Design review of the part built by this model. Coordinates are the model's own, in mm. A direction names the side the tool comes from. Round coordinates to 2 decimals unless told otherwise and drop trailing zeros. Order: outer loops, then holes, each group sorted by start corner. A loop starts at its lowest first (then second) coordinate and runs counter-clockwise, first axis right, second up. Notation, with made-up numbers: (-17.75, -3) - (36.25, -3) arc R28 ccw to (36.25, 34) - close; hole circle Ø3 at (-35.5, 7.5). An arc over 180 degrees is marked (long way). Write item = value, one per line.
from build123d import *

# Parameters (mm, degrees)
BOSS_EXTRUDE1_DEPTH = 60
BOSS_EXTRUDE2_DEPTH = 1.5
CUT_EXTRUDE1_DEPTH  = 122.5
FILLET1_R           = 2
SKETCH4_R           = 1
CUT_EXTRUDE2_DEPTH  = 122.5
SKETCH5_W           = 20.552185026
SKETCH5_H           = 10
CUT_EXTRUDE3_DEPTH  = 66.5
CHAMFER2_SIZE       = 4


with BuildPart() as part:
    # Sketch1 → Boss-Extrude1 (new body)
    with BuildSketch(Plane(origin=(0, 0, 0), x_dir=(1, 0, 0), z_dir=(0, 1, 0))):
        Polygon((-25.683056898, 37.455662838), (17.724607753, 43.304991821), (29.01282847, -40.464497095), (-14.394836181, -46.313826078), align=None)
        Polygon((-23.996173554, 36.169418466), (16.438363381, 41.618108478), (27.325945127, -39.178252723), (-13.108591809, -44.626942734), align=None, mode=Mode.SUBTRACT)
    extrude(amount=BOSS_EXTRUDE1_DEPTH)

    # Sketch2 → Boss-Extrude2 (add)
    with BuildSketch(Plane(origin=(0, 60, 0), x_dir=(1, 0, 0), z_dir=(0, 1, 0))):
        Polygon((-25.683056898, 37.455662838), (-14.394836181, -46.313826078), (29.01282847, -40.464497095), (17.724607753, 43.304991821), align=None)
    extrude(amount=BOSS_EXTRUDE2_DEPTH)

    # Sketch3 → Cut-Extrude1 (cut)
    with BuildSketch(Plane(origin=(5.87291271, 0, 43.582678665), x_dir=(0.991042572, 0, -0.133546324), z_dir=(0.133546324, 0, 0.991042572))):
        with BuildLine():
            Line((21.449063315, 0), (21.449063315, 10))
            ThreePointArc((21.449063315, 10), (18.520131127, 17.071067812), (11.449063315, 20))
            Line((11.449063315, 20), (-8.550936685, 20))
            ThreePointArc((-8.550936685, 20), (-15.622004497, 17.071067812), (-18.550936685, 10))
            Line((-18.550936685, 10), (-18.550936685, 0))
            Line((-18.550936685, 0), (21.449063315, 0))
        make_face()
        with BuildLine():
            ThreePointArc((11.449063315, 20), (18.520131127, 17.071067812), (21.449063315, 10))
            Line((21.449063315, 10), (21.449063315, 0))
            Line((21.449063315, 0), (21.849063315, 0))
            Line((21.849063315, 0), (21.849063315, 10))
            ThreePointArc((21.849063315, 10), (18.802973839, 17.353910524), (11.449063315, 20.4))
            Line((11.449063315, 20.4), (-8.550936685, 20.4))
            ThreePointArc((-8.550936685, 20.4), (-15.90484721, 17.353910524), (-18.950936685, 10))
            Line((-18.950936685, 10), (-18.950936685, 0))
            Line((-18.950936685, 0), (-18.550936685, 0))
            Line((-18.550936685, 0), (-18.550936685, 10))
            ThreePointArc((-18.550936685, 10), (-15.622004497, 17.071067812), (-8.550936685, 20))
            Line((-8.550936685, 20), (11.449063315, 20))
        make_face()
    extrude(amount=-CUT_EXTRUDE1_DEPTH, mode=Mode.SUBTRACT)

    # Fillet1
    fillet1_edges = [part.edges().sort_by_distance(p)[0] for p in [
        (17.724607753, 30.75, -43.304991821),
        (-25.683056898, 30.75, -37.455662838),
        (-14.394836181, 30.75, 46.313826078),
        (29.01282847, 30.75, 40.464497095),
    ]]
    fillet(fillet1_edges, radius=FILLET1_R)

    # Sketch4 → Cut-Extrude2 (cut)
    with BuildSketch(Plane(origin=(23.13991576, 0, -3.11818157), x_dir=(-0.133546324, 0, -0.991042572), z_dir=(0.991042572, 0, -0.133546324))):
        with Locations((-24.013280796, 5)):
            Circle(SKETCH4_R)
        with Locations((20.586719204, 5)):
            Circle(SKETCH4_R)
    extrude(amount=-CUT_EXTRUDE2_DEPTH, mode=Mode.SUBTRACT)

    # Sketch5 → Cut-Extrude3 (cut)
    with BuildSketch(Plane(origin=(-20.267748891, 0, 2.731147413), x_dir=(0.133546324, 0, 0.991042572), z_dir=(-0.991042572, 0, 0.133546324))):
        with Locations((0, 5)):
            Rectangle(SKETCH5_W, SKETCH5_H)
    extrude(amount=-CUT_EXTRUDE3_DEPTH, mode=Mode.SUBTRACT)

    # Chamfer2
    chamfer2_edges = [part.edges().sort_by_distance(p)[0] for p in [
        (21.024299453, 10, -13.202066981),
        (-20.89680134, 10, -7.553057484),
        (23.768968209, 10, 7.166023327),
        (-18.152132584, 10, 12.815032824),
    ]]
    chamfer(chamfer2_edges, length=CHAMFER2_SIZE)


solid = part.part
Item 1: The part is to be moulded in two halves that separate along Y. For faces 1 (the face through (25.487, 5.3, 19.833)), 2 (the face through (7, 20.4, 43)), 3 (the face through (-13.91, 31.18, 45.64)), say which applies: +Y half, -Y half, draft (parallel to the pull), parting line (faces both ways), or undercut.
Data:
face_1 = undercut
face_2 = -Y half
face_3 = draft
Item 2: For faces 4 (the face through (7.392, 40.206, 41.864)), 5 (the face through (24.49, 17.27, 40.33)), 6 (the face through (-4, 20.4, -40)), list the 3-axis set-ups (+Z, -Z, +X, -X, +Y, -Y) from which the entire face can be reached by the end or side of a thin tool; tool diameter is ignored.
Data:
face_4 = -Y
face_5 = +Z, -Y
face_6 = -Z, -Y
Item 3: Take a section at B-B, the plane y = 18.5. State the section outline as (x, z) points.
Data:
outline = (-25.42, -35.47) arc R2 ccw to (-23.7, -37.72) - (-19.83, -38.24) - (-19.63, -36.76) - (-24, -36.17) - (-13.11, 44.63) - (-8.74, 44.04) - (-8.54, 45.52) - (-12.41, 46.05) arc R2 ccw to (-14.66, 44.33) - close; (11.87, -42.52) - (15.74, -43.04) arc R2 ccw to (17.99, -41.32) - (28.75, 38.48) arc R2 ccw to (27.03, 40.73) - (23.16, 41.25) - (22.96, 39.77) - (27.33, 39.18) - (16.44, -41.62) - (12.07, -41.03) - close
Item 4: Take a section at A-A, the plane y = 37. State the section outline as (x, z) points.
Data:
outline = (-25.42, -35.47) arc R2 ccw to (-23.7, -37.72) - (15.74, -43.04) arc R2 ccw to (17.99, -41.32) - (28.75, 38.48) arc R2 ccw to (27.03, 40.73) - (-12.41, 46.05) arc R2 ccw to (-14.66, 44.33) - close; hole (-24, -36.17) - (16.44, -41.62) - (27.33, 39.18) - (-13.11, 44.63) - close
Item 5: Take a section at D-D, the plane x = 4. State the section outline as (y, z) points.
Data:
outline = (20.4, -41.46) - (61.5, -41.46) - (61.5, 43.84) - (20.4, 43.84) - (20.4, 42.32) - (60, 42.32) - (60, -39.94) - (20.4, -39.94) - close
Item 6: Take a section at C-C, the plane z = -31.5. State the section outline as (x, y) points, and give its area (3 significant figures).
Data:
outline = (-24.88, 0) - (-23.37, 0) - (-23.37, 60) - (17.8, 60) - (17.8, 0) - (19.32, 0) - (19.32, 61.5) - (-24.88, 61.5) - close
area = 248 mm2
Item 7: For line 1 along Y through (x, z) = (7.5, 31.5); line 2 along X through (y, z) = (47, -3); line 3 along X through (y, z) = (38.5, 32.5), list the stretches that pass through material, from the lowest coordinate up. Write a range as [from, to].
Data:
line_1 = [60, 61.5]
line_2 = [-21.04, -19.53], [21.64, 23.16]
line_3 = [-16.26, -14.74], [26.43, 27.94]
Item 8: Insertion check: P1, Ø1, axis at x = 17.5, y = 39.5, coming from the +Z side; P2, Ø4, axis at x = 1.5, z = 36, coming from the -Y side; P3, Ø1.2, axis at x = -3, z = -39.5, coming from the -Y side. Each pin has a flat end and moves straight along its axis. Give the tip position at first contact, or say it passes through.
Data:
P1 = 42.08
P2 = 60
P3 = 20.4
